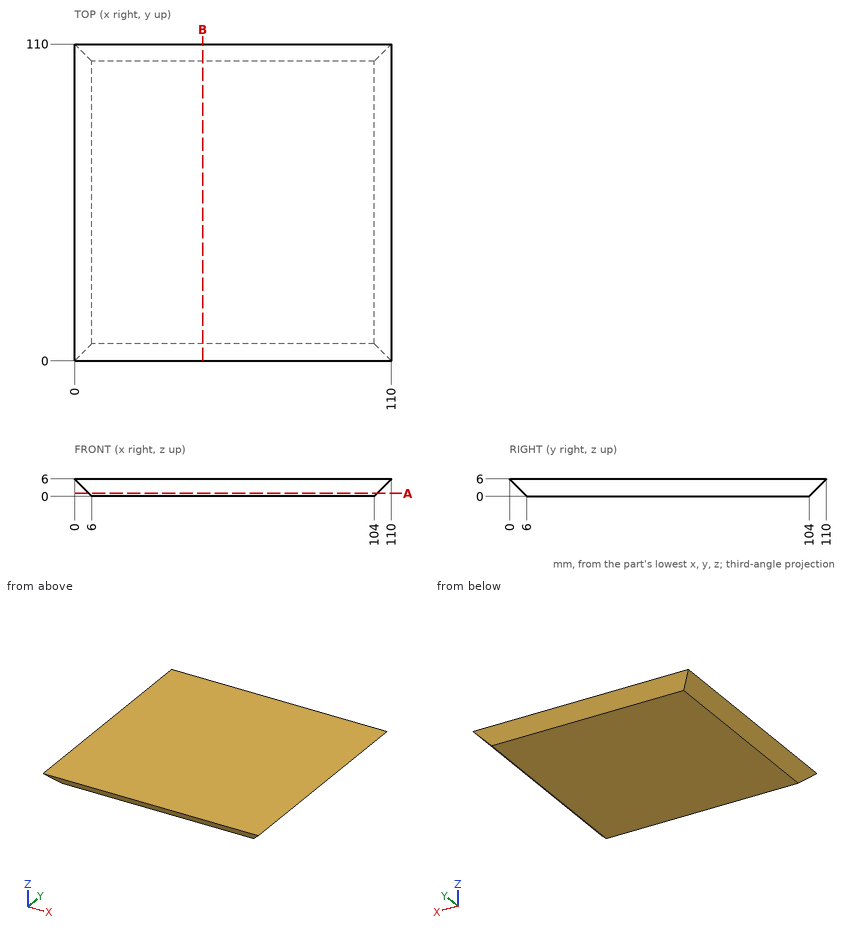
For this review, use the dimensioned drawing (mm, ordinates from the lowest corner) and the shaded views. Round coordinates to 2 decimals unless told otherwise and drop trailing zeros. Order: outer loops, then holes, each group sorted by start corner. A loop starts at its lowest first (then second) coordinate and runs counter-clockwise, first axis right, second up.
1) Consider section B-B (x = 44.5). State the section outline as (y, z) points.
The answers:
outline: (0, 6) - (6, 0) - (104, 0) - (110, 6) - close
2) For L1, parallel to X at y = 32.5, z = 4.75; L2, parallel to X at y = 11.5, z = 3.5; L3, parallel to Y at x = 60, z = 5, list the stretches that pass through material, from the lowest coordinate up.
The answers:
L1: x = 1.25 to 108.75
L2: x = 2.5 to 107.5
L3: y = 1 to 109
3) Clearance check with flat-ended pins moving along their axes: pin 1 Ø1 at (y, z) = (48, 4.5) entering from +X; pin 2 Ø1.5 at (x, z) = (68.5, 2) entering from +Y; pin 3 Ø3 at (y, z) = (66.5, 0.5) entering from -X. State where each tip first meets the part, or that it passes through.
The answers:
pin 1: stops at x = 109
pin 2: stops at y = 106.75
pin 3: stops at x = 4
4) Consider section A-A (z = 1). State the section outline as (x, y) points, plus the area to 3 significant figures.
The answers:
outline: (5, 5) - (105, 5) - (105, 105) - (5, 105) - close
area: 10,000 mm2
